Geometry: final body of the model. Coordinates: model frame, mm. A direction names the side the tool comes from. Give positions to 0.01 mm unless a question says otherwise; leave off trailing zeros. Write each loop counter-clockwise with the first axis right and the second up, starting at its lowest first coordinate (ties: lowest second). Pieces come first, ordered by that corner, then holes. Notation, with made-up numbers: M -35,17 L -1,17 A12 ccw -1,28 Z; hole C 7.25,33.5 d11. An arc over 180 degrees is marked long. Answer as a JSON object with one key per item and string values.
from build123d import *

# Parameters (mm, degrees)
F0_R     = 41.5
F0_R_2   = 2.5
F0_R_3   = 26.85
F0_R_4   = 22.5
F1_DEPTH = 8
F2_DEPTH = 2
F3_R     = 2
F3_R_2   = 22.5
F3_R_3   = 11.5
F4_DEPTH = 16
F5_R     = 15.5
F5_R_2   = 11.5
F6_DEPTH = 3


with BuildPart() as f1:
    # F0 (on Top) → F1 (new body)
    with BuildSketch(Plane.XY):
        Circle(F0_R)
        with Locations((-7.5753864878, -34.1703602492)):
            Circle(F0_R_2, mode=Mode.SUBTRACT)
        with Locations((-33.3800932762, -10.5247029826)):
            Circle(F0_R_2, mode=Mode.SUBTRACT)
        with Locations((25.8047067884, -23.6456572665)):
            Circle(F0_R_2, mode=Mode.SUBTRACT)
        with Locations((-25.8047067884, 23.6456572665)):
            Circle(F0_R_2, mode=Mode.SUBTRACT)
        Circle(F0_R_3, mode=Mode.SUBTRACT)
        with Locations((33.3800932762, 10.5247029826)):
            Circle(F0_R_2, mode=Mode.SUBTRACT)
        with Locations((7.5753864878, 34.1703602492)):
            Circle(F0_R_2, mode=Mode.SUBTRACT)
        Circle(F0_R_3)
        Circle(F0_R_4, mode=Mode.SUBTRACT)
    extrude(amount=F1_DEPTH)

    # F0 (on Top) → F2 (cut)
    with BuildSketch(Plane.XY):
        Circle(F0_R_3)
        Circle(F0_R_4, mode=Mode.SUBTRACT)
    extrude(amount=F2_DEPTH, mode=Mode.SUBTRACT)

    # F3 (on face) → F4 (join)
    with BuildSketch(Plane.XY.offset(8)):
        with BuildLine():
            ThreePointArc((31.1379786303, -20.8968008752), (35.8742539897, -10.9219000491), (37.5, 0))
            ThreePointArc((37.5, 0), (37.3878227586, 2.8983977242), (37.0519621671, 5.7794549545))
            ThreePointArc((37.051962167, 5.7794549545), (27.6577915717, 8.7204681856), (33.6661497309, 16.5178800787))
            ThreePointArc((33.6661497309, 16.5178800787), (25.3346327856, 27.6479001304), (13.5208262729, 34.977667974))
            ThreePointArc((13.5208262729, 34.977667974), (13.5617308945, 34.5749348961), (13.5753864878, 34.1703602492))
            ThreePointArc((13.5753864878, 34.1703602492), (5.8847198032, 28.4134820881), (2.5281711006, 37.4146809539))
            ThreePointArc((2.5281711006, 37.414680954), (-11.2764674814, 35.7643856531), (-23.5311358942, 29.1982130195))
            ThreePointArc((-23.5311358942, 29.1982130195), (-20.8226677798, 26.9892013918), (-19.8047067884, 23.6456572665))
            ThreePointArc((-19.8047067884, 23.6456572665), (-24.390428006, 17.8147211903), (-31.1379786303, 20.8968008752))
            ThreePointArc((-31.1379786303, 20.8968008752), (-36.611100267, 8.1164855227), (-37.051962167, -5.7794549545))
            ThreePointArc((-37.0519621671, -5.7794549545), (-30.7372929948, -5.1380893272), (-27.3800932762, -10.5247029826))
            ThreePointArc((-27.3800932762, -10.5247029826), (-29.2398238845, -14.8673023614), (-33.6661497309, -16.5178800787))
            ThreePointArc((-33.6661497309, -16.5178800787), (-25.3346327856, -27.6479001304), (-13.5208262729, -34.977667974))
            ThreePointArc((-13.5208262729, -34.977667974), (-7.9799611347, -28.1840158425), (-1.5753864878, -34.1703602492))
            ThreePointArc((-1.5753864878, -34.1703602492), (-1.8185083267, -35.8610269338), (-2.5281711006, -37.4146809539))
            ThreePointArc((-2.5281711006, -37.414680954), (11.2764674814, -35.7643856531), (23.5311358942, -29.1982130195))
            ThreePointArc((23.5311358942, -29.1982130195), (21.3810427675, -19.5921160209), (31.1379786303, -20.8968008752))
        make_face()
        with Locations((-22.5166604984, -13)):
            Circle(F3_R, mode=Mode.SUBTRACT)
        with Locations((0, -26)):
            Circle(F3_R, mode=Mode.SUBTRACT)
        with Locations((22.5166604984, -13)):
            Circle(F3_R, mode=Mode.SUBTRACT)
        with Locations((-22.5166604984, 13)):
            Circle(F3_R, mode=Mode.SUBTRACT)
        Circle(F3_R_2, mode=Mode.SUBTRACT)
        with Locations((22.5166604984, 13)):
            Circle(F3_R, mode=Mode.SUBTRACT)
        with Locations((0, 26)):
            Circle(F3_R, mode=Mode.SUBTRACT)
        Circle(F3_R_2)
        Circle(F3_R_3, mode=Mode.SUBTRACT)
    extrude(amount=F4_DEPTH)

    # F5 (on face) → F6 (join)
    with BuildSketch(Plane.XY.offset(24)):
        Circle(F5_R)
        Circle(F5_R_2, mode=Mode.SUBTRACT)
    extrude(amount=F6_DEPTH)


solid = f1.part
1) Cut plane D-D on z = 25.75. Return loops of the section in (x, y).
Geometry check:
{"outline": "C 0,0 d31; hole C 0,0 d23"}
2) Contact query for flat-ended pins moving along their axis: P1, Ø3, axis at x = 23, y = 12.5, coming from the +Z side; P2, Ø1, axis at y = -29.5, z = 24, coming from the +X side; P3, Ø2, axis at y = 32, z = 23, coming from the -X side; P4, Ø6.5, axis at x = 0, y = -26, coming from the -Z side. Output: stop coordinate, or through.
Geometry check:
{"P1": "stops at z = 24", "P2": "stops at x = 23.53", "P3": "stops at x = -21.1", "P4": "stops at z = 0"}
3) Line query: line 1 (Y direction, x = 0, z = 16.25); line 2 (X direction, y = 11.5, z = 4.25); line 3 (Y direction, x = 0, z = 1.55). Output: solid intervals per line, ascending. Write a range as from..to.
Geometry check:
{"line 1": "y = -37.5..-28, -24..-11.5, 11.5..24, 28..37.5", "line 2": "x = -39.87..-19.34, 19.34..31.08, 35.68..39.87", "line 3": "y = -41.5..-26.85, 26.85..41.5"}
4) Cut plane C-C on x = -9. Return loops of the section in (y, z), and give its area (3 significant figures).
Geometry check:
{"outline": "M -40.51,0 L -36.22,0 L -36.22,8 L -40.51,8 Z; M -32.12,0 L -25.3,0 L -25.3,2 L -20.62,2 L -20.62,8 L -7.16,8 L -7.16,27 L -12.62,27 L -12.62,24 L -28.34,24 L -28.34,8 L -32.12,8 Z; M 7.16,8 L 20.62,8 L 20.62,2 L 25.3,2 L 25.3,0 L 40.51,0 L 40.51,8 L 36.4,8 L 36.4,24 L 12.62,24 L 12.62,27 L 7.16,27 Z", "area": "1,110 mm2"}
5) Cut plane B-B on z = 13.75. Return loops of the section in (x, y).
Geometry check:
{"outline": "M -37.05,-5.78 A6 cw long -33.67,-16.52 A37.5 ccw -13.52,-34.98 A6 cw long -2.53,-37.41 A37.5 ccw 23.53,-29.2 A6 cw long 31.14,-20.9 A37.5 ccw 37.05,5.78 A6 cw long 33.67,16.52 A37.5 ccw 13.52,34.98 A6 cw long 2.53,37.41 A37.5 ccw -23.53,29.2 A6 cw long -31.14,20.9 A37.5 ccw Z; hole C -22.52,-13 d4; hole C -22.52,13 d4; hole C 0,0 d23; hole C 0,-26 d4; hole C 0,26 d4; hole C 22.52,-13 d4; hole C 22.52,13 d4"}
6) Pull-direction query (Y, two-part tool) for faces 6 (the flat face through (16, 1, 24)), 7 (the cylindrical face through (-35.878, -10.415, 3.944)), 8 (the cylindrical face through (-36.568, 8.308, 15.888)); classes: pulls with the +Y half, pulls with the -Y half, needs draft (parallel to the pull), parting line crosses it, or undercut.
Geometry check:
{"face 6": "needs draft", "face 7": "undercut", "face 8": "parting line crosses it"}
7) Set-up query: faces 1 (the cylindrical face through (0, 24, 16)), 2 (the cylindrical face through (-25.479, -27.515, 15.888)), 3 (the cylindrical face through (10.382, -19.961, 4.958)), 4 (the flat face through (0, 12, 27)), 5 (the flat face through (-1, -27, 0)). Return all of +Z, -Z, +X, -X, +Y, -Y with unobstructed straight access to the full face (end or side cutting, diameter ignored); none if empty.
Geometry check:
{"face 1": "+Z", "face 2": "+Z, -X, -Y", "face 3": "-Z", "face 4": "+Z, +X, -X, +Y, -Y", "face 5": "-Z, +X, -X, +Y, -Y"}
